Could you check a few things on this model? Use its own coordinates, in mm. A direction names the side the tool comes from. Round coordinates to 2 decimals unless told otherwise and drop trailing zeros. Loops run counter-clockwise (first coordinate to the right, second up) from the corner with the lowest first, then second, coordinate; pieces in that order, holes last. Notation, with made-up numbers: (67, -17.5) - (110, -17.5) arc R22 cw to (110, -1.5) - close; hole circle Ø6 at (-1, 64.25). An arc over 180 degrees is marked (long way). Use one line per item in the form item = value.
```python
from build123d import *

# Parameters (mm, degrees)
SKETCH1_R           = 4
BOSS_EXTRUDE1_DEPTH = 7
SKETCH2_R           = 4
BOSS_EXTRUDE2_DEPTH = 4
SKETCH3_R           = 1.9
CUT_EXTRUDE1_DEPTH  = 4


with BuildPart() as part:
    # Sketch1 → Boss-Extrude1 (new body)
    with BuildSketch(Plane.XY):
        Circle(SKETCH1_R)
        Polygon((-1.6, 0), (-1.6, 2.6), (1.6, 2.6), (1.6, -2.6), (-1.6, -2.6), align=None, mode=Mode.SUBTRACT)
    extrude(amount=BOSS_EXTRUDE1_DEPTH)

    # Sketch2 → Boss-Extrude2 (add)
    with BuildSketch(Plane.XY.offset(7)):
        Circle(SKETCH2_R)
    extrude(amount=BOSS_EXTRUDE2_DEPTH)

    # Sketch3 → Cut-Extrude1 (cut)
    with BuildSketch(Plane.XY.offset(11)):
        Circle(SKETCH3_R)
    extrude(amount=-CUT_EXTRUDE1_DEPTH, mode=Mode.SUBTRACT)


solid = part.part
```
1. Please list where these lines run through material, in increasing order: line 1 along Y through (x, z) = (0, 9.85); line 2 along Y through (x, z) = (0, 3.5); line 3 along X through (y, z) = (-1.25, 2.25).
Solution:
line_1 = -4 to -1.9, 1.9 to 4
line_2 = -4 to -2.6, 2.6 to 4
line_3 = -3.8 to -1.6, 1.6 to 3.8
2. If we section it at A-A, the plane y = 0: Write out the boundary of the cut face in (x, z).
Solution:
outline = (-4, 0) - (-1.6, 0) - (-1.6, 7) - (-1.9, 7) - (-1.9, 11) - (-4, 11) - close; (1.6, 0) - (4, 0) - (4, 11) - (1.9, 11) - (1.9, 7) - (1.6, 7) - close
3. If we section it at D-D, the plane z = 8.75: Write out the boundary of the cut face in (x, y), plus the area to 3 significant figures.
Solution:
outline = circle Ø8 at (0, 0); hole circle Ø3.8 at (0, 0)
area = 38.9 mm^2
4. If we section it at C-C, the plane z = 6.75: Write out the boundary of the cut face in (x, y), plus the area to 3 significant figures.
Solution:
outline = circle Ø8 at (0, 0); hole (-1.6, -2.6) - (1.6, -2.6) - (1.6, 2.6) - (-1.6, 2.6) - close
area = 33.6 mm^2
5. For P1, Ø1.5, axis at y = 1.5, z = 9, coming from the +X side; P2, Ø1.7, axis at x = 0, y = 1.5, coming from the -Z side; P3, Ø2, axis at x = 2.5, z = 3.5, coming from the -Y side, each with a flat end and sliding along its axis, tell me the tip position at first contact or that it passes through.
Solution:
P1 = 3.93
P2 = 7
P3 = -3.71
6. We'd pull the mould along X, two halves only. Please class faces 3 (the face through (-1.9, 0.08, 9.03)), 4 (the face through (-0.867, -3.905, 5.423)), 5 (the face through (2, 0, 0)): +X half, -X half, draft (parallel to the pull), parting line (faces both ways), or undercut.
Solution:
face_3 = undercut
face_4 = parting line
face_5 = draft
7. On a 3-axis mill with a long thin cutter (end or side, diameter ignored), from which of +Z, -Z, +X, -X, +Y, -Y can I reach the whole of each face in a straight line? I mean faces 1 (the face through (2, -1, 11)), 2 (the face through (0, -2.2, 7)). Say none if no direction works.
Solution:
face_1 = +Z, +X, -X, +Y, -Y
face_2 = -Z
8. If we section it at B-B, the plane x = 0: Write out the boundary of the cut face in (y, z), plus the area to 3 significant figures.
Solution:
outline = (-4, 0) - (-2.6, 0) - (-2.6, 7) - (-1.9, 7) - (-1.9, 11) - (-4, 11) - close; (1.9, 7) - (2.6, 7) - (2.6, 0) - (4, 0) - (4, 11) - (1.9, 11) - close
area = 36.4 mm^2
